from build123d import *

# Parameters (mm, degrees)
F1_DEPTH = 1.778
F2_R     = 0.577688
F2_R_2   = 0.582255
F3_DEPTH = 15.3416
F4_R     = 5.08


with BuildPart() as f1:
    # F0 (on Top) → F1 (new body, symmetric)
    with BuildSketch(Plane.XY):
        Polygon((-25.4, -42.175161), (25.4, -42.175161), (25.4, -29.790713), (15.341625, -29.790713), (15.341625, -15.554283), (25.4, -15.554283), (25.4, 17.656827), (15.341625, 17.656827), (15.341625, 31.893248), (25.4, 31.893248), (25.4, 42.175161), (-25.4, 42.175161), (-25.4, 31.893248), (-15.341633, 31.893248), (-15.341633, 17.65682), (-25.4, 17.65682), (-25.4, -15.554283), (-15.341625, -15.554283), (-15.341625, -29.790713), (-25.4, -29.790713), align=None)
    extrude(amount=F1_DEPTH, both=True)

    # F2 (on Right) → F3 (join, symmetric)
    with BuildSketch(Plane.YZ):
        with BuildLine():
            Line((-27.829766, 1.773621), (-17.552791, 1.808458))
            ThreePointArc((-17.552791, 1.808458), (-22.703696, 5.454035), (-27.829766, 1.773621))
        make_face()
        with Locations((-22.68527, 3.27162)):
            Circle(F2_R, mode=Mode.SUBTRACT)
        with BuildLine():
            Line((20.001708, 1.808458), (30.278683, 1.773621))
            ThreePointArc((30.278683, 1.773621), (25.152562, 5.439228), (20.001708, 1.808458))
        make_face()
        with Locations((25.134111, 3.27162)):
            Circle(F2_R_2, mode=Mode.SUBTRACT)
    extrude(amount=F3_DEPTH, both=True)

    # F4
    f4_edges = [f1.edges().sort_by_distance(p)[0] for p in [
        (25.4, -42.175161, 0),
        (-25.4, -42.175161, 0),
        (-25.4, -29.790713, 0),
        (-25.4, -15.554283, 0),
        (-25.4, 17.65682, 0),
        (-25.4, 31.893248, 0),
        (-25.4, 42.175161, 0),
        (25.4, 42.175161, 0),
        (25.4, 17.656827, 0),
        (25.4, 31.893248, 0),
        (25.4, -29.790713, 0),
        (25.4, -15.554283, 0),
    ]]
    fillet(f4_edges, radius=F4_R)


solid = f1.part
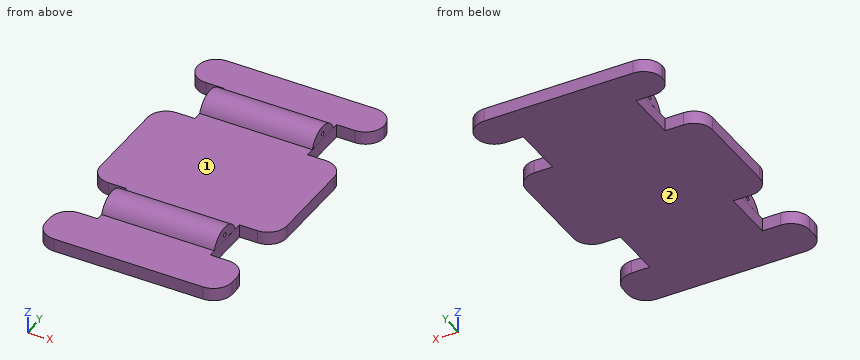
Could you check a few things on this model? Use its own coordinates, in mm. Face numbers are marked on the shaded views. Give positions to 0.01 mm unless a question says otherwise; leave off trailing zeros. Write each loop counter-clockwise with the first axis right and the second up, starting at its lowest first coordinate (ties: lowest second). Pieces come first, ordered by that corner, then holes. Notation, with made-up numbers: (-11, -11.5) -> (15, -11.5) arc R28 cw to (15, 9.5) -> close; hole circle Ø7 at (-15, 78). An arc over 180 degrees is marked (long way). Write each question's results on one line, items separated by ' | '. Start each with the question number.
Q1. Suppose I cut it at C-C, the plane y = -25. List the corners of the cut face in (x, z) for me, and give its area (3 significant figures).
Q2. Suppose I cut it at B-B, the plane x = 22. List the corners of the cut face in (y, z) for me.
Q3. I'm going to push flat-ended pins straight in: pin 1 Ø1.8 at (y, z) = (26.5, 0) entering from -X; pin 2 Ø3 at (x, z) = (11.5, 4) entering from +Y; pin 3 Ø1 at (x, y) = (3.5, 25.5) entering from +Z. Where does each tip first touch, or does it pass through?
Q4. Suppose I cut it at A-A, the plane x = 5. List the corners of the cut face in (y, z) for me.
Q5. I need wall thicknesses on probe 1 along Y at (x, z) = (18, 0.75); probe 2 along Y at (x, z) = (11, 3.25); probe 3 along X at (y, z) = (-22, -1). Which ranges of each line are inside material? Lowest first, please.
Q6. We'd pull the mould along Y, two halves only. Please class the marked faces 1 and 2: +Y half, -Y half, draft (parallel to the pull), parting line (faces both ways), or undercut.
Outcome:
1) outline: (-15.34, -1.78) -> (15.34, -1.78) -> (15.34, 1.78) -> (-15.34, 1.78) -> close; (-15.34, 1.78) -> (15.34, 1.78) -> (15.34, 4.94) -> (-15.34, 4.94) -> close | area: 206 mm2
2) outline: (-41.89, -1.78) -> (-30.08, -1.78) -> (-30.08, 1.78) -> (-41.89, 1.78) -> close; (-15.27, -1.78) -> (17.37, -1.78) -> (17.37, 1.78) -> (-15.27, 1.78) -> close; (32.18, -1.78) -> (41.89, -1.78) -> (41.89, 1.78) -> (32.18, 1.78) -> close
3) pin 1: x = -15.34 | pin 2: y = 29.97 | pin 3: z = 5.44
4) outline: (-42.18, -1.78) -> (42.18, -1.78) -> (42.18, 1.78) -> (30.28, 1.78) arc R5.44 ccw to (20, 1.81) -> (28.99, 1.78) -> (-26.54, 1.78) -> (-17.55, 1.81) arc R5.44 ccw to (-27.83, 1.78) -> (-42.18, 1.78) -> close; hole circle Ø1.16 at (-22.69, 3.27); hole circle Ø1.16 at (25.13, 3.27)
5) probe 1: -42.18 to -29.79, -15.55 to 17.66, 31.89 to 42.18 | probe 2: -27.06 to -23.26, -22.11 to -18.31, 20.77 to 24.55, 25.72 to 29.5 | probe 3: -15.34 to 15.34
6) face 1: undercut | face 2: draft
